```python
from build123d import *

# Parameters (mm, degrees)
BOSS_EXTRUDE1_DEPTH = 25
SKETCH1_3_W         = 25
SKETCH1_3_H         = 12
BOSS_EXTRUDE2_DEPTH = 50
SKETCH1_4_W         = 25
SKETCH1_4_H         = 12
BOSS_EXTRUDE3_DEPTH = 38


with BuildPart() as part:
    # Sketch1 → Boss-Extrude1 (new body)
    with BuildSketch(Plane.XY):
        Polygon((-25, 12), (0, 12), (0, 37), (-20, 37), (-55, 12), (-50, 12), align=None)
    extrude(amount=BOSS_EXTRUDE1_DEPTH)

    # Sketch1_3 → Boss-Extrude2 (add)
    with BuildSketch(Plane.XY):
        Polygon((-50, 0), (-50, 12), (-55, 12), (-75, 12), (-75, 0), align=None)
        with Locations((-12.5, 6)):
            Rectangle(SKETCH1_3_W, SKETCH1_3_H)
    extrude(amount=BOSS_EXTRUDE2_DEPTH)

    # Sketch1_4 → Boss-Extrude3 (add)
    with BuildSketch(Plane.XY):
        with Locations((-37.5, 6)):
            Rectangle(SKETCH1_4_W, SKETCH1_4_H)
    extrude(amount=BOSS_EXTRUDE3_DEPTH)


solid = part.part
```
For this review, take the finished solid that the model builds, in its own axes (mm). A direction names the side the tool comes from. Coordinates: 2 decimals unless noted, no trailing zeros. Order: outer loops, then holes, each group sorted by start corner. A loop starts at its lowest first (then second) coordinate and runs counter-clockwise, first axis right, second up. Notation, with made-up numbers: (53.5, -2.5) - (82.5, -2.5) arc R19 ccw to (82.5, 12.5) - close; hole circle Ø4 at (51, 29.25). An arc over 180 degrees is marked (long way). Answer as a JSON object with one key per item and string values. Group by question number.
1. For faces 1 (the flat face through (0, 14, 19)), 2 (the flat face through (-50, 6, 44)), 3 (the flat face through (-38, 0, 25)), 4 (the flat face through (-46, 12, 30)), 5 (the flat face through (-22, 22, 25)), list the 3-axis set-ups (+Z, -Z, +X, -X, +Y, -Y) from which the entire face can be reached by the end or side of a thin tool; tool diameter is ignored.
2. We need section A-A on y = 7. State the section outline as (x, z) points.
3. We need section C-C on z = 19. State the section outline as (x, y) points, then the cut area to 3 significant figures.
4. Clearance check with flat-ended pins moving along their axes: P1, Ø12.5, axis at x = -39, y = 30.5, coming from the +Z side; P2, Ø2, axis at y = 6, z = 33, coming from the +X side; P3, Ø12, axis at y = 33, z = 9, coming from the -X side; P4, Ø3.5, axis at x = -40.5, y = 4.5, coming from the +Z side. State where each tip first meets the part, or that it passes through.
5. We need section D-D on x = -58.5. State the section outline as (y, z) points.
6. For probe 1 along Y at (x, z) = (-67.5, 32); probe 2 along Z at (x, y) = (-10.5, 19); probe 3 along X at (y, z) = (20, 24), list the stretches that pass through material, from the lowest coordinate up.
7. We need section B-B on x = -23.5. State the section outline as (y, z) points.
8. The part is to be moulded in two halves that separate along X. For faces 6 (the flat face through (-25, 6, 44)), 7 (the flat face through (-38, 6, 38)), 8 (the flat face through (-37.26, 24.67, 12.32)), 9 (the flat face through (-13, 6, 50)), say which applies: pulls with the +X half, pulls with the -X half, needs draft (parallel to the pull), parting line crosses it, or undercut.
Final values:
{
 "1": {"face 1": "+Z, -Z, +X, +Y, -Y", "face 2": "+Z, +Y, -Y", "face 3": "+Z, -Z, +X, -X, -Y", "face 4": "+Z, -X, +Y", "face 5": "+Z, +X, -X, +Y"},
 "2": {"outline": "(-75, 0) - (0, 0) - (0, 50) - (-25, 50) - (-25, 38) - (-50, 38) - (-50, 50) - (-75, 50) - close"},
 "3": {"outline": "(-75, 0) - (0, 0) - (0, 37) - (-20, 37) - (-55, 12) - (-75, 12) - close", "area": "1,840 mm²"},
 "4": {"P1": "z = 25", "P2": "x = 0", "P3": "x = -34", "P4": "z = 38"},
 "5": {"outline": "(0, 0) - (12, 0) - (12, 50) - (0, 50) - close"},
 "6": {"probe 1": "0 to 12", "probe 2": "0 to 25", "probe 3": "-43.8 to 0"},
 "7": {"outline": "(0, 0) - (34.5, 0) - (34.5, 25) - (12, 25) - (12, 50) - (0, 50) - close"},
 "8": {"face 6": "undercut", "face 7": "undercut", "face 8": "pulls with the -X half", "face 9": "needs draft"}
}
